Check sheet for the drawn part. Datum: minimum x, y, z corner. Units: mm. A direction names the side the tool comes from. Give positions to 0.01 mm unless a question says otherwise; leave off trailing zeros. Order: outer loops, then holes, each group sorted by start corner. A loop starts at its lowest first (then second) coordinate and runs counter-clockwise, first axis right, second up.
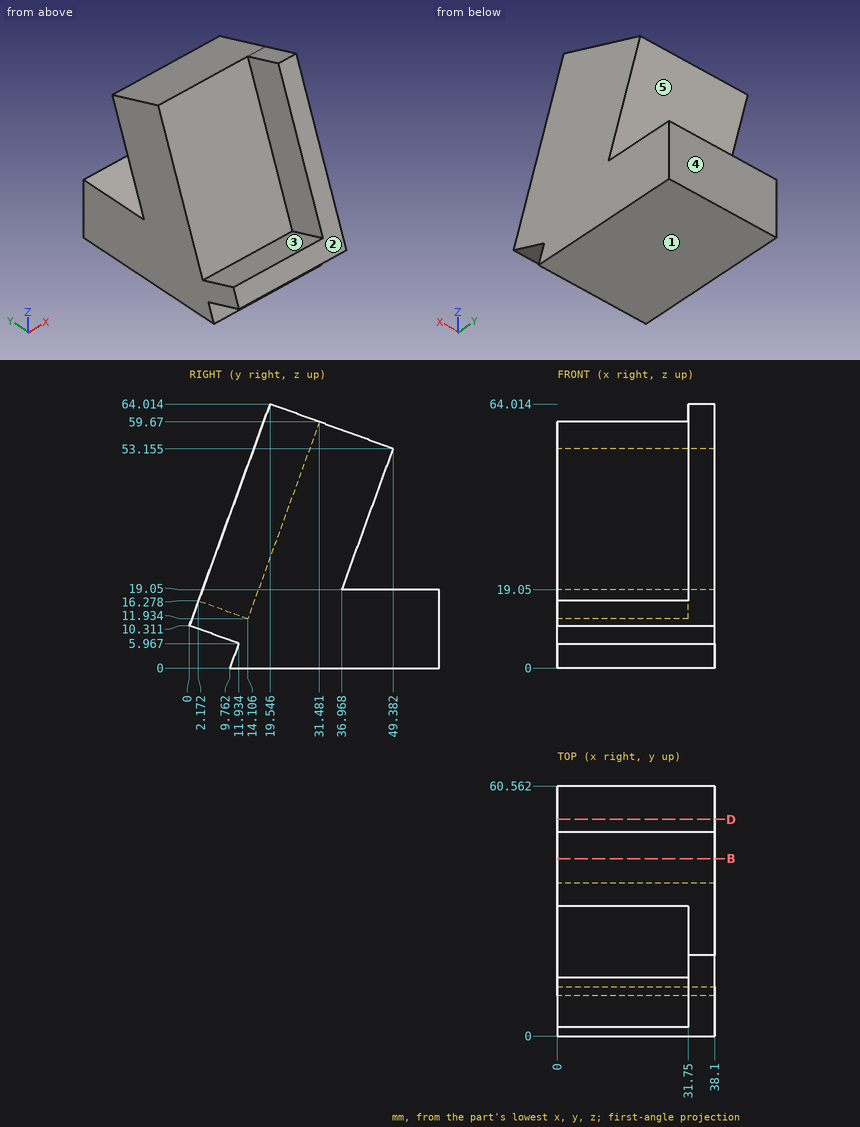
(1) Set-up check for the marked faces 4 and 5: record each of +Z, -Z, +X, -X, +Y, -Y from which the full face is reachable in a straight line by a thin tool's end or side.
Solved:
face 4: +Z, -Z, +X, -X, +Y
face 5: +X, -X, +Y
(2) Go/stop test with flat-tipped pins: pin 1 (7 mm diameter, centred on x = 14.5, y = 51, fed in from +Z); pin 2 (12 mm diameter, centred on x = 21, z = 37.5, fed in from +Y); pin 3 (2 mm diameter, centred on x = 13.5, y = 44, fed in from +Z). Record where each tip stops, or that it passes through.
Solved:
pin 1: stops at z = 53.84
pin 2: stops at y = 45.87
pin 3: stops at z = 55.48
(3) Scan lines: line 1 (X direction, y = 31, z = 59.5); line 2 (Z direction, x = 36, y = 53); line 3 (Y direction, x = 19.5, z = 26) (1 decimal). Record each from-to range of solid material in increasing order.
Solved:
line 1: x = 31.75 to 38.1
line 2: z = 0 to 19.05
line 3: y = 19.2 to 39.5
(4) Section check B-B, the plane y = 43. Enter the section's corners in (x, z).
Solved:
outline: (0, 0) - (38.1, 0) - (38.1, 19.05) - (0, 19.05) - close; (0, 35.62) - (38.1, 35.62) - (38.1, 55.48) - (0, 55.48) - close
(5) Release check for a two-part mould opening along Y. For the marked faces 1, 2 and 3 record: pulls with the +Y half, pulls with the -Y half, needs draft (parallel to the pull), parting line crosses it, or undercut.
Solved:
face 1: needs draft
face 2: pulls with the -Y half
face 3: undercut
(6) Section check D-D, the plane y = 52.5. Enter the section's corners in (x, z).
Solved:
outline: (0, 0) - (38.1, 0) - (38.1, 19.05) - (0, 19.05) - close
